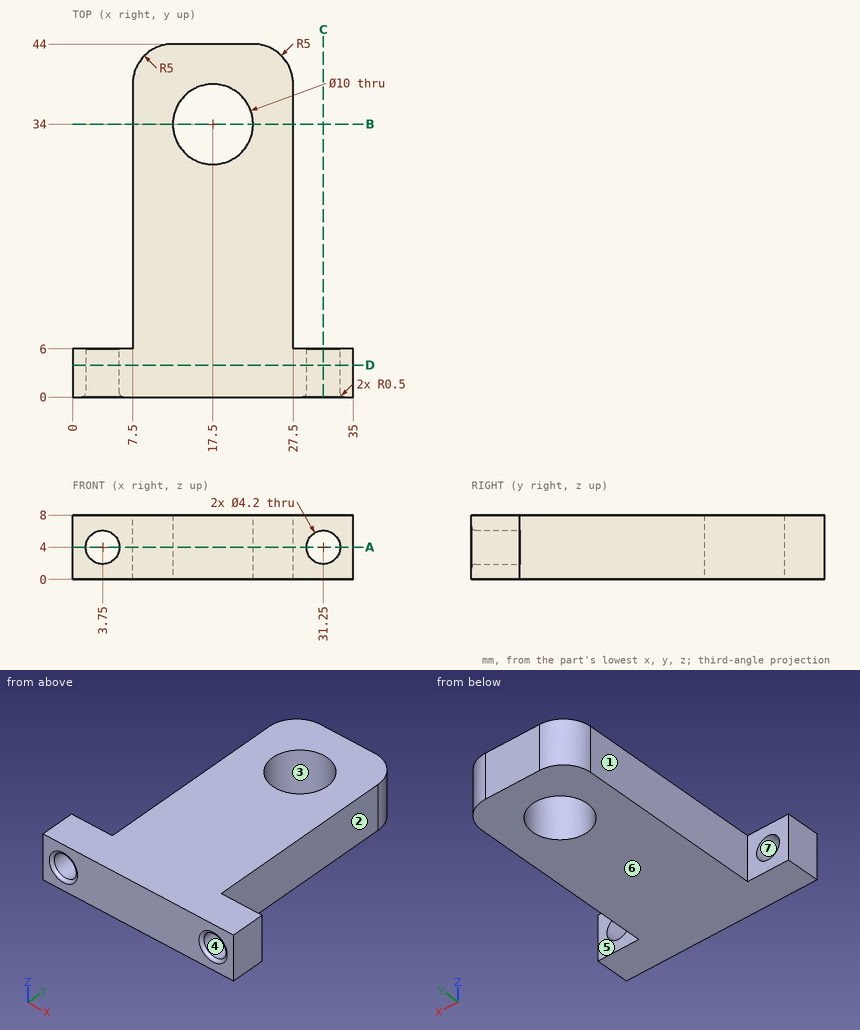
Verification items for this drawing (mm, ordinates from the low corner). A direction names the side the tool comes from. Round coordinates to 2 decimals unless told otherwise and drop trailing zeros. Order: outer loops, then holes, each group sorted by start corner. A loop starts at its lowest first (then second) coordinate and runs counter-clockwise, first axis right, second up. Notation, with made-up numbers: (84, 9) - (123, 9) arc R32 ccw to (123, 35) - close; hole circle Ø4 at (-23.75, 57.5). An arc over 180 degrees is marked (long way). Use CSV: the item, a comma, the result in double quotes. Start each with the question number.
1) Section check C-C, the plane x = 31.25. Record the cut outline in (y, z), plus the area to 3 significant figures.
2) Mould release check, pull along Z, two halves, no side actions. Record for the marked faces 4, 5, 6 and 7: +Z half, -Z half, draft (parallel to the pull), parting line (faces both ways), or undercut.
3) Section check A-A, the plane z = 4. Record the cut outline in (x, y).
4) Thickness scan on L1, parallel to Y at x = 17.5, z = 2.5; L2, parallel to Y at x = 13.5, z = 2; L3, parallel to X at y = 10.5, z = 5.5. Record the ranges inside material, lowest first.
5) Access from +Z, -Z, +X, -X, +Y, -Y to the whole of each face (thin tool, end or side, straight path). Record for the marked faces 1, 2 and 3.
6) Section check B-B, the plane y = 34. Record the cut outline in (x, z).
7) Go/stop test with flat-tipped pins: P1, Ø4, axis at x = 30, z = 3.5, coming from the +Y side; P2, Ø1, axis at y = 11, z = 2.5, coming from the +X side; P3, Ø3, axis at y = 10, z = 4.5, coming from the -X side. Record where each tip stops, or that it passes through.
8) Section check D-D, the plane y = 4. Record the cut outline in (x, z).
Answers:
1,outline,"(0, 0) - (6, 0) - (6, 1.9) - (0.5, 1.9) arc R0.5 ccw to (0, 1.4) - close; (0, 6.6) arc R0.5 ccw to (0.5, 6.1) - (6, 6.1) - (6, 8) - (0, 8) - close"
1,area,"22.7 mm²"
2,face 4,"undercut"
2,face 5,"draft"
2,face 6,"-Z half"
2,face 7,"undercut"
3,outline,"(0, 0) - (1.15, 0) arc R0.5 ccw to (1.65, 0.5) - (1.65, 6) - (0, 6) - close; (5.85, 0.5) arc R0.5 ccw to (6.35, 0) - (28.65, 0) arc R0.5 ccw to (29.15, 0.5) - (29.15, 6) - (27.5, 6) - (27.5, 39) arc R5 ccw to (22.5, 44) - (12.5, 44) arc R5 ccw to (7.5, 39) - (7.5, 6) - (5.85, 6) - close; (33.35, 0.5) arc R0.5 ccw to (33.85, 0) - (35, 0) - (35, 6) - (33.35, 6) - close; hole circle Ø10 at (17.5, 34)"
4,L1,"y = 0 to 29, 39 to 44"
4,L2,"y = 0 to 31, 37 to 44"
4,L3,"x = 7.5 to 27.5"
5,face 1,"+Z, -Z, -X, +Y"
5,face 2,"+Z, -Z, +X, +Y"
5,face 3,"+Z, -Z"
6,outline,"(7.5, 0) - (12.5, 0) - (12.5, 8) - (7.5, 8) - close; (22.5, 0) - (27.5, 0) - (27.5, 8) - (22.5, 8) - close"
7,P1,"stops at y = 6"
7,P2,"stops at x = 27.5"
7,P3,"stops at x = 7.5"
8,outline,"(0, 0) - (35, 0) - (35, 8) - (0, 8) - close; hole circle Ø4.2 at (3.75, 4); hole circle Ø4.2 at (31.25, 4)"
